Part model, mm, in its own coordinate system. Coordinates: 2 decimals unless noted, no trailing zeros. Loops run counter-clockwise (first coordinate to the right, second up) from the corner with the lowest first, then second, coordinate; pieces in that order, holes last. Notation, with made-up numbers: M 25,6.5 L 43,6.5 A31 cw 43,45.5 Z; hole C 79,13.25 d6. An arc over 180 degrees is marked long. Answer as a JSON object with one key per item and string values. Group by question number.
1. Drill centre lines: L1, parallel to X at y = 1.2, z = -100; L2, parallel to Z at x = -12, y = 1.15; L3, parallel to Z at x = -6, y = 1.3. Where is each one in solid material? Low to high.
2. Saw through at A-A on x = -11. Write the cut outline in (y, z) (3 decimals).
3. Saw through at D-D on z = -109. Write the cut outline in (x, y) (3 decimals).
4. Drop flat-ended pins along their axis: pin 1 Ø1.5 at (y, z) = (1.5, 47) entering from +X; pin 2 Ø5 at (x, z) = (2.5, -47) entering from -Y; pin 3 Ø3 at (x, z) = (0, -126.25) entering from -Y. Give the stop position or say it passes through.
5. Saw through at C-C on y = 0.7. Write the cut outline in (x, z).
6. Saw through at B-B on z = 91.5. Write the cut outline in (x, y) (3 decimals).
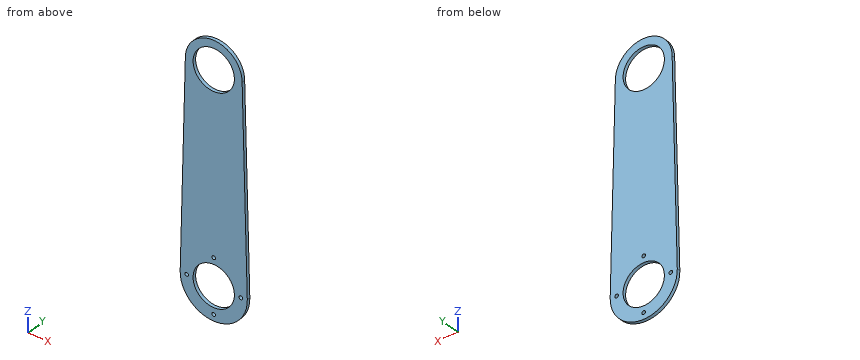
from build123d import *

# Parameters (mm, degrees)
BOSS_EXTRUDE1_DEPTH     = 3.175
SKETCH2_R               = 20
CUT_EXTRUDE1_DEPTH      = 137.464576448
ESQUISSE2_R             = 1.75
ENL_V_MAT_EXTRU_1_DEPTH = 137.464576448


with BuildPart() as part:
    # Sketch1 → Boss-Extrude1 (new body)
    with BuildSketch(Plane(origin=(0, 0, 0), x_dir=(1, 0, 0), z_dir=(0, 1, 0))):
        with BuildLine():
            Line((-27.5, -100), (-32.489807083, 99.186098474))
            ThreePointArc((-32.489807083, 99.186098474), (0, 132.5), (32.489807083, 99.186098474))
            Line((32.489807083, 99.186098474), (27.5, -100))
            ThreePointArc((27.5, -100), (0, -127.5), (-27.5, -100))
        make_face()
    extrude(amount=BOSS_EXTRUDE1_DEPTH)

    # Sketch2 → Cut-Extrude1 (cut, through all)
    with BuildSketch(Plane(origin=(0, 3.175, 0), x_dir=(1, 0, 0), z_dir=(0, 1, 0))):
        with Locations(Location((0, -100, 0), (0, 0, 270))):
            Circle(SKETCH2_R)
        with Locations(Location((0, 100, 0), (0, 0, 270))):
            Circle(SKETCH2_R)
    extrude(amount=-CUT_EXTRUDE1_DEPTH, mode=Mode.SUBTRACT)

    # Esquisse2 → Enlèv. mat.-Extru.1 (cut, through all)
    with BuildSketch(Plane(origin=(0, 3.175, 0), x_dir=(1, 0, 0), z_dir=(0, 1, 0))):
        with Locations(Location((0, 73.75, 0), (0, 0, 270))):
            Circle(ESQUISSE2_R)
        with Locations(Location((26.25, 100, 0), (0, 0, 270))):
            Circle(ESQUISSE2_R)
        with Locations(Location((0, 126.25, 0), (0, 0, 270))):
            Circle(ESQUISSE2_R)
        with Locations(Location((-26.25, 100, 0), (0, 0, 270))):
            Circle(ESQUISSE2_R)
    extrude(amount=-ENL_V_MAT_EXTRU_1_DEPTH, mode=Mode.SUBTRACT)


solid = part.part
Outcome:
{
 "1": {"L1": "x = -32.5 to -28, -24.5 to -20, 20 to 24.5, 28 to 32.5", "L2": "z = -130.2 to -116, -84 to 84, 116 to 124.74", "L3": "z = -131.94 to -119.08, -80.92 to 80.92, 119.08 to 126.84"},
 "2": {"outline": "M 0,-130.582 L 3.175,-130.582 L 3.175,-116.703 L 0,-116.703 Z; M 0,-83.297 L 3.175,-83.297 L 3.175,83.297 L 0,83.297 Z; M 0,116.703 L 3.175,116.703 L 3.175,125.204 L 0,125.204 Z"},
 "3": {"outline": "M -31.229,0 L -17.861,0 L -17.861,3.175 L -31.229,3.175 Z; M 17.861,0 L 31.229,0 L 31.229,3.175 L 17.861,3.175 Z"},
 "4": {"pin 1": "stops at x = 28.85", "pin 2": "stops at y = 0", "pin 3": "passes through"},
 "5": {"outline": "M -32.49,-99.19 A32.5 ccw long 32.49,-99.19 L 27.5,100 A27.5 ccw -27.5,100 Z; hole C -26.25,-100 d3.5; hole C 0,-100 d40; hole C 0,100 d40; hole C 0,-126.25 d3.5; hole C 0,-73.75 d3.5; hole C 26.25,-100 d3.5"},
 "6": {"outline": "M -27.713,0 L -18.104,0 L -18.104,3.175 L -27.713,3.175 Z; M 18.104,0 L 27.713,0 L 27.713,3.175 L 18.104,3.175 Z"}
}
